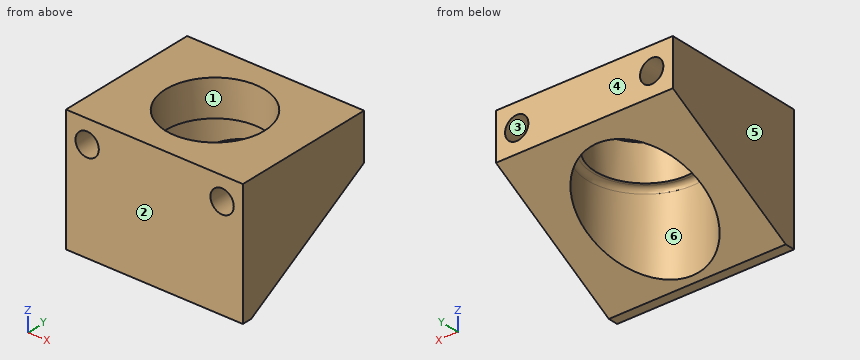
from build123d import *

# Parameters (mm, degrees)
SKETCH1_W          = 54.102
SKETCH1_H          = 44.45
SKETCH1_R          = 15.1003
EXTRUDE1_DEPTH     = 38.1
CUT_EXTRUDE1_DEPTH = 55.102
SKETCH3_R          = 17.526
CUT_EXTRUDE2_DEPTH = 26.9748
FILLET1_R          = 1.524
HOLE1_D            = 7.1374
HOLE1_DEPTH        = 44.45


with BuildPart() as part:
    # Sketch1 → Extrude1 (new body)
    with BuildSketch(Plane.XY):
        with Locations((0, 22.225)):
            Rectangle(SKETCH1_W, SKETCH1_H)
        with Locations((0, 22.225)):
            Circle(SKETCH1_R, mode=Mode.SUBTRACT)
    extrude(amount=-EXTRUDE1_DEPTH)

    # Sketch2 → Cut-Extrude1 (cut, through all)
    with BuildSketch(Plane(origin=(27.051, 0, 0), x_dir=(0, 0, -1), z_dir=(1, 0, 0))):
        Polygon((14.224, 44.45), (38.1, 3.048), (38.1, 44.45), align=None)
    extrude(amount=-CUT_EXTRUDE1_DEPTH, mode=Mode.SUBTRACT)

    # Sketch3 → Cut-Extrude2 (cut)
    with BuildSketch(Plane(origin=(0, 0, -38.1), x_dir=(-1, 0, 0), z_dir=(0, 0, -1))):
        with Locations(Location((0, 22.225, 0), (0, 0, 270))):  # turned: the seam where the file's is
            Circle(SKETCH3_R)
    extrude(amount=-CUT_EXTRUDE2_DEPTH, mode=Mode.SUBTRACT)

    # Fillet1
    fillet1_edges = [part.edges().sort_by_distance(p)[0] for p in [
        (0, 39.751, -11.1252),
    ]]
    fillet(fillet1_edges, radius=FILLET1_R)

    # Hole1
    with Locations(Plane(origin=(0, 44.45, 0), x_dir=(-1, 0, 0), z_dir=(0, 1, 0))):
        with Locations((20.574, -7.112), (-20.701, -7.112)):
            Hole(HOLE1_D / 2, depth=HOLE1_DEPTH)


solid = part.part
Can you work these out from the model? Positions are in its coordinate system, mm. Face numbers are marked on the shaded views. A direction names the side the tool comes from. Give positions to 0.01 mm unless a question says otherwise; leave off trailing zeros. Order: outer loops, then holes, each group sorted by start corner. A loop starts at its lowest first (then second) coordinate and runs counter-clockwise, first axis right, second up. Notation, with made-up numbers: M 77.5,37.25 L 105.5,37.25 A24 cw 105.5,57.25 Z; hole C -33,57 d1. An arc over 180 degrees is marked long. Use one line per item in the form item = value.
Item 1: If I drill on line 1 along Y through (x, z) = (0, -3.75); line 2 along X through (y, z) = (22.5, -24.5); line 3 along X through (y, z) = (25, -14), over which ranges is the centre line in solid material (lowest first)? Write a range as [from, to].
Values follow:
line_1 = [0, 7.12], [37.33, 44.45]
line_2 = [-27.05, -17.52], [17.52, 27.05]
line_3 = [-27.05, -17.3], [17.3, 27.05]
Item 2: If we section it at D-D, the plane y = 41.5: Write out the boundary of the cut face in (x, z).
Values follow:
outline = M -27.05,-15.93 L 27.05,-15.93 L 27.05,0 L -27.05,0 Z; hole C -20.57,-7.11 d7.14; hole C 20.7,-7.11 d7.14
Item 3: If we section it at C-C, the plane y = 15: Count the separate pieces of the cut face and the enclosed holes in it, and give its area (3 significant figures).
Values follow:
separate_pieces = 2
enclosed_holes = 2
area = 673 mm^2
Item 4: If we section it at B-B, the plane x = 19: Write out the boundary of the cut face in (y, z), and give its area (3 significant figures).
Values follow:
outline = M 0,-38.1 L 3.05,-38.1 L 44.45,-14.22 L 44.45,-10.25 L 0,-10.25 Z; M 0,-3.97 L 44.45,-3.97 L 44.45,0 L 0,0 Z
area = 920 mm^2
Item 5: Thinking about a two-plate mould opening in Y: for the marked faces 1, 2, 3 and 4, which applies, pulls with the +Y half, pulls with the -Y half, needs draft (parallel to the pull), parting line crosses it, or undercut?
Values follow:
face_1 = undercut
face_2 = pulls with the -Y half
face_3 = needs draft
face_4 = pulls with the +Y half
Item 6: If we section it at A-A, the plane z = -9.5: Write out the boundary of the cut face in (x, y) (3 decimals).
Values follow:
outline = M -27.051,0 L -23.226,0 L -23.226,44.45 L -27.051,44.45 Z; M -17.922,0 L 18.049,0 L 18.049,44.45 L -17.922,44.45 Z; M 23.353,0 L 27.051,0 L 27.051,44.45 L 23.353,44.45 Z; hole C 0,22.225 d30.201
Item 7: For the marked faces 5 and 6, which set-ups out of +Z, -Z, +X, -X, +Y, -Y let a thin tool reach every point of the face, with its end or its side?
Values follow:
face_5 = +Z, -Z, -X, +Y, -Y
face_6 = -Z
